from build123d import *

# Parameters (mm, degrees)
BOSS_EXTRUDE1_DEPTH      = 1.3
BOSS_EXTRUDE2_DEPTH      = 3.8
BOSS_EXTRUDE3_DEPTH      = 5.7
SKETCH4_R                = 0.5
CUT_EXTRUDE1_DEPTH       = 5.7
LPATTERN1_COUNT          = 6
LPATTERN1_PITCH          = 3
MIRROR1_COPY_1_SKETCH_R  = 0.5
MIRROR1_COPY_1_DEPTH     = 5.7
MIRROR1_COPY_2_SKETCH_R  = 0.5
MIRROR1_COPY_2_DEPTH     = 5.7
MIRROR1_COPY_3_SKETCH_R  = 0.5
MIRROR1_COPY_3_DEPTH     = 5.7
MIRROR1_COPY_4_SKETCH_R  = 0.5
MIRROR1_COPY_4_DEPTH     = 5.7
MIRROR1_COPY_5_SKETCH_R  = 0.5
MIRROR1_COPY_5_DEPTH     = 5.7
MIRROR2_COPY_1_SKETCH_R  = 0.5
MIRROR2_COPY_1_DEPTH     = 5.7
MIRROR2_COPY_2_SKETCH_R  = 0.5
MIRROR2_COPY_2_DEPTH     = 5.7
MIRROR2_COPY_3_SKETCH_R  = 0.5
MIRROR2_COPY_3_DEPTH     = 5.7
MIRROR2_COPY_4_SKETCH_R  = 0.5
MIRROR2_COPY_4_DEPTH     = 5.7
MIRROR2_COPY_5_SKETCH_R  = 0.5
MIRROR2_COPY_5_DEPTH     = 5.7
MIRROR2_COPY_6_SKETCH_R  = 0.5
MIRROR2_COPY_6_DEPTH     = 5.7
MIRROR2_COPY_7_SKETCH_R  = 0.5
MIRROR2_COPY_7_DEPTH     = 5.7
MIRROR2_COPY_8_SKETCH_R  = 0.5
MIRROR2_COPY_8_DEPTH     = 5.7
MIRROR2_COPY_9_SKETCH_R  = 0.5
MIRROR2_COPY_9_DEPTH     = 5.7
MIRROR2_COPY_10_SKETCH_R = 0.5
MIRROR2_COPY_10_DEPTH    = 5.7
MIRROR2_COPY_11_SKETCH_R = 0.5
MIRROR2_COPY_11_DEPTH    = 5.7
MIRROR2_COPY_12_SKETCH_R = 0.5
MIRROR2_COPY_12_DEPTH    = 5.7
MIRROR2_COPY_13_SKETCH_R = 0.5
MIRROR2_COPY_13_DEPTH    = 5.7
SKETCH5_R                = 1.55
CUT_EXTRUDE2_DEPTH       = 28.864942132


with BuildPart() as part:
    # Sketch1 → Boss-Extrude1 (new body)
    with BuildSketch(Plane.XY):
        with BuildLine():
            Line((-25.05, -6.25), (25.05, -6.25))
            ThreePointArc((25.05, -6.25), (26.110660172, -5.810660172), (26.55, -4.75))
            Line((26.55, -4.75), (26.55, 4.75))
            ThreePointArc((26.55, 4.75), (26.110660172, 5.810660172), (25.05, 6.25))
            Line((25.05, 6.25), (-25.05, 6.25))
            ThreePointArc((-25.05, 6.25), (-26.110660172, 5.810660172), (-26.55, 4.75))
            Line((-26.55, 4.75), (-26.55, -4.75))
            ThreePointArc((-26.55, -4.75), (-26.110660172, -5.810660172), (-25.05, -6.25))
        make_face()
    extrude(amount=BOSS_EXTRUDE1_DEPTH)

    # Sketch2 → Boss-Extrude2 (add)
    with BuildSketch(Plane(origin=(0, 0, 0), x_dir=(-1, 0, 0), z_dir=(0, 0, -1))):
        with BuildLine():
            Line((-18.7, -5.5), (18.7, -5.5))
            ThreePointArc((18.7, -5.5), (20.114213562, -4.914213562), (20.7, -3.5))
            Line((20.7, -3.5), (20.7, 3.5))
            ThreePointArc((20.7, 3.5), (20.114213562, 4.914213562), (18.7, 5.5))
            Line((18.7, 5.5), (-18.7, 5.5))
            ThreePointArc((-18.7, 5.5), (-20.114213562, 4.914213562), (-20.7, 3.5))
            Line((-20.7, 3.5), (-20.7, -3.5))
            ThreePointArc((-20.7, -3.5), (-20.114213562, -4.914213562), (-18.7, -5.5))
        make_face()
    extrude(amount=BOSS_EXTRUDE2_DEPTH)

    # Sketch3 → Boss-Extrude3 (add)
    with BuildSketch(Plane.XY.offset(1.3)):
        with BuildLine():
            Line((-17.25, -4.1), (17.25, -4.1))
            ThreePointArc((17.25, -4.1), (18.664213562, -3.514213562), (19.25, -2.1))
            Line((19.25, -2.1), (19.25, 2.1))
            ThreePointArc((19.25, 2.1), (18.664213562, 3.514213562), (17.25, 4.1))
            Line((17.25, 4.1), (-17.25, 4.1))
            ThreePointArc((-17.25, 4.1), (-18.664213562, 3.514213562), (-19.25, 2.1))
            Line((-19.25, 2.1), (-19.25, -2.1))
            ThreePointArc((-19.25, -2.1), (-18.664213562, -3.514213562), (-17.25, -4.1))
        make_face()
    extrude(amount=BOSS_EXTRUDE3_DEPTH)

    # Sketch4 → Cut-Extrude1 (cut)
    with BuildSketch(Plane.XY.offset(7)):
        with Locations((0, 2)):
            Circle(SKETCH4_R)
    cut_extrude1 = extrude(amount=-CUT_EXTRUDE1_DEPTH, mode=Mode.SUBTRACT)

    # LPattern1: Cut-Extrude1 ×6
    with Locations(*[(i * LPATTERN1_PITCH, 0, 0) for i in range(1, LPATTERN1_COUNT)]):
        add(cut_extrude1, mode=Mode.SUBTRACT)

    # Mirror1: Cut-Extrude1 across plane
    add(cut_extrude1.mirror(Plane.ZX), mode=Mode.SUBTRACT)

    # Mirror1 copy 1 sketch → Mirror1 copy 1 (cut)
    with BuildSketch(Plane(origin=(3, 0, 7), x_dir=(1, 0, 0), z_dir=(0, 0, 1))):
        with Locations((0, -2)):
            Circle(MIRROR1_COPY_1_SKETCH_R)
    extrude(amount=-MIRROR1_COPY_1_DEPTH, mode=Mode.SUBTRACT)

    # Mirror1 copy 2 sketch → Mirror1 copy 2 (cut)
    with BuildSketch(Plane(origin=(6, 0, 7), x_dir=(1, 0, 0), z_dir=(0, 0, 1))):
        with Locations((0, -2)):
            Circle(MIRROR1_COPY_2_SKETCH_R)
    extrude(amount=-MIRROR1_COPY_2_DEPTH, mode=Mode.SUBTRACT)

    # Mirror1 copy 3 sketch → Mirror1 copy 3 (cut)
    with BuildSketch(Plane(origin=(9, 0, 7), x_dir=(1, 0, 0), z_dir=(0, 0, 1))):
        with Locations((0, -2)):
            Circle(MIRROR1_COPY_3_SKETCH_R)
    extrude(amount=-MIRROR1_COPY_3_DEPTH, mode=Mode.SUBTRACT)

    # Mirror1 copy 4 sketch → Mirror1 copy 4 (cut)
    with BuildSketch(Plane(origin=(12, 0, 7), x_dir=(1, 0, 0), z_dir=(0, 0, 1))):
        with Locations((0, -2)):
            Circle(MIRROR1_COPY_4_SKETCH_R)
    extrude(amount=-MIRROR1_COPY_4_DEPTH, mode=Mode.SUBTRACT)

    # Mirror1 copy 5 sketch → Mirror1 copy 5 (cut)
    with BuildSketch(Plane(origin=(15, 0, 7), x_dir=(1, 0, 0), z_dir=(0, 0, 1))):
        with Locations((0, -2)):
            Circle(MIRROR1_COPY_5_SKETCH_R)
    extrude(amount=-MIRROR1_COPY_5_DEPTH, mode=Mode.SUBTRACT)

    # Mirror2 copy 1 sketch → Mirror2 copy 1 (cut)
    with BuildSketch(Plane(origin=(-3, 0, 7), x_dir=(-1, 0, 0), z_dir=(0, 0, 1))):
        with Locations((0, -2)):
            Circle(MIRROR2_COPY_1_SKETCH_R)
    extrude(amount=-MIRROR2_COPY_1_DEPTH, mode=Mode.SUBTRACT)

    # Mirror2 copy 2 sketch → Mirror2 copy 2 (cut)
    with BuildSketch(Plane(origin=(-6, 0, 7), x_dir=(-1, 0, 0), z_dir=(0, 0, 1))):
        with Locations((0, -2)):
            Circle(MIRROR2_COPY_2_SKETCH_R)
    extrude(amount=-MIRROR2_COPY_2_DEPTH, mode=Mode.SUBTRACT)

    # Mirror2 copy 3 sketch → Mirror2 copy 3 (cut)
    with BuildSketch(Plane(origin=(-9, 0, 7), x_dir=(-1, 0, 0), z_dir=(0, 0, 1))):
        with Locations((0, -2)):
            Circle(MIRROR2_COPY_3_SKETCH_R)
    extrude(amount=-MIRROR2_COPY_3_DEPTH, mode=Mode.SUBTRACT)

    # Mirror2 copy 4 sketch → Mirror2 copy 4 (cut)
    with BuildSketch(Plane(origin=(-12, 0, 7), x_dir=(-1, 0, 0), z_dir=(0, 0, 1))):
        with Locations((0, -2)):
            Circle(MIRROR2_COPY_4_SKETCH_R)
    extrude(amount=-MIRROR2_COPY_4_DEPTH, mode=Mode.SUBTRACT)

    # Mirror2 copy 5 sketch → Mirror2 copy 5 (cut)
    with BuildSketch(Plane(origin=(-15, 0, 7), x_dir=(-1, 0, 0), z_dir=(0, 0, 1))):
        with Locations((0, -2)):
            Circle(MIRROR2_COPY_5_SKETCH_R)
    extrude(amount=-MIRROR2_COPY_5_DEPTH, mode=Mode.SUBTRACT)

    # Mirror2 copy 6 sketch → Mirror2 copy 6 (cut)
    with BuildSketch(Plane(origin=(0, 0, 7), x_dir=(-1, 0, 0), z_dir=(0, 0, 1))):
        with Locations((0, -2)):
            Circle(MIRROR2_COPY_6_SKETCH_R)
    extrude(amount=-MIRROR2_COPY_6_DEPTH, mode=Mode.SUBTRACT)

    # Mirror2 copy 7 sketch → Mirror2 copy 7 (cut)
    with BuildSketch(Plane(origin=(0, 0, 7), x_dir=(-1, 0, 0), z_dir=(0, 0, 1))):
        with Locations((0, 2)):
            Circle(MIRROR2_COPY_7_SKETCH_R)
    extrude(amount=-MIRROR2_COPY_7_DEPTH, mode=Mode.SUBTRACT)

    # Mirror2 copy 8 sketch → Mirror2 copy 8 (cut)
    with BuildSketch(Plane(origin=(-3, 0, 7), x_dir=(-1, 0, 0), z_dir=(0, 0, 1))):
        with Locations((0, 2)):
            Circle(MIRROR2_COPY_8_SKETCH_R)
    extrude(amount=-MIRROR2_COPY_8_DEPTH, mode=Mode.SUBTRACT)

    # Mirror2 copy 9 sketch → Mirror2 copy 9 (cut)
    with BuildSketch(Plane(origin=(-6, 0, 7), x_dir=(-1, 0, 0), z_dir=(0, 0, 1))):
        with Locations((0, 2)):
            Circle(MIRROR2_COPY_9_SKETCH_R)
    extrude(amount=-MIRROR2_COPY_9_DEPTH, mode=Mode.SUBTRACT)

    # Mirror2 copy 10 sketch → Mirror2 copy 10 (cut)
    with BuildSketch(Plane(origin=(-9, 0, 7), x_dir=(-1, 0, 0), z_dir=(0, 0, 1))):
        with Locations((0, 2)):
            Circle(MIRROR2_COPY_10_SKETCH_R)
    extrude(amount=-MIRROR2_COPY_10_DEPTH, mode=Mode.SUBTRACT)

    # Mirror2 copy 11 sketch → Mirror2 copy 11 (cut)
    with BuildSketch(Plane(origin=(-12, 0, 7), x_dir=(-1, 0, 0), z_dir=(0, 0, 1))):
        with Locations((0, 2)):
            Circle(MIRROR2_COPY_11_SKETCH_R)
    extrude(amount=-MIRROR2_COPY_11_DEPTH, mode=Mode.SUBTRACT)

    # Mirror2 copy 12 sketch → Mirror2 copy 12 (cut)
    with BuildSketch(Plane(origin=(-15, 0, 7), x_dir=(-1, 0, 0), z_dir=(0, 0, 1))):
        with Locations((0, 2)):
            Circle(MIRROR2_COPY_12_SKETCH_R)
    extrude(amount=-MIRROR2_COPY_12_DEPTH, mode=Mode.SUBTRACT)

    # Mirror2 copy 13 sketch → Mirror2 copy 13 (cut)
    with BuildSketch(Plane(origin=(0, 0, 7), x_dir=(-1, 0, 0), z_dir=(0, 0, 1))):
        with Locations((0, -2)):
            Circle(MIRROR2_COPY_13_SKETCH_R)
    extrude(amount=-MIRROR2_COPY_13_DEPTH, mode=Mode.SUBTRACT)

    # Sketch5 → Cut-Extrude2 (cut, through all)
    with BuildSketch(Plane.XY.offset(1.3)):
        with Locations((23.75, 0)):
            Circle(SKETCH5_R)
    cut_extrude2 = extrude(amount=-CUT_EXTRUDE2_DEPTH, mode=Mode.SUBTRACT)

    # Mirror3: Cut-Extrude2 across plane
    add(cut_extrude2.mirror(Plane(origin=(0, 0, 0), x_dir=(0, 0, 1), z_dir=(1, 0, 0))), mode=Mode.SUBTRACT)


solid = part.part
Read the model definition and answer for the solid it produces. Units are mm, in the model's axes. A direction names the side the tool comes from. Round coordinates to 2 decimals unless told otherwise and drop trailing zeros. Loops run counter-clockwise (first coordinate to the right, second up) from the corner with the lowest first, then second, coordinate; pieces in that order, holes last.
Q1. Consider probe 1 along Y at (x, z) = (-15, 4.05); probe 2 along Z at (x, y) = (-22, -3); probe 3 along Y at (x, z) = (2, 6). Determine where each line is inside the solid, lowest interval first.
Q2. Section D-D on x = -18 is taken. Write down the section's boundary in (y, z), and give its area (3 significant figures).
Q3. Section B-B on y = 0 is taken. Write down the section's boundary in (x, z), and give its area (3 significant figures).
Q4. Section A-A on z = 4.75 is taken. Give the number of separate pieces and of enclosed holes in the cut face, and give its area (3 significant figures).
Q5. Determine the mould class of faces 4 (the face through (20.7, 0, -2)), 5 (the face through (-20.13, 4.9, -1.87)), 6 (the face through (2.6, 2.3, 4.2)) for opening direction X: released by +X, released by -X, zero draft, split by the parting line, or undercut.
Q6. Which of the six approach directions +Z, -Z, +X, -X, +Y, -Y give full straight-line access (tool end or side, diameter ignored) to faces 1 (the face through (18.68, 3.5, 4.11)), 2 (the face through (-12, 2, 1.3)), 3 (the face through (0, 6, 0))?
Q7. Section C-C on x = 13.5 is taken. Write down the section's boundary in (y, z).
Q8. Each of these flat-tipped pins is pushed along its axis until it touches: pin 1 (3 mm diameter, centred on x = -8.5, z = 4.5, fed in from +Y); pin 2 (3 mm diameter, centred on x = -4, z = -2, fed in from -Y); pin 3 (0.8 mm diameter, centred on x = 9, y = 2, fed in from +Z). Where does it stop, or does it pass through?
Output:
1. probe 1: y = -4.1 to -2.5, -1.5 to 1.5, 2.5 to 4.1
1. probe 2: z = 0 to 1.3
1. probe 3: y = -4.1 to 4.1
2. outline: (-6.25, 0) - (-5.5, 0) - (-5.5, -3.8) - (5.5, -3.8) - (5.5, 0) - (6.25, 0) - (6.25, 1.3) - (3.95, 1.3) - (3.95, 7) - (-3.95, 7) - (-3.95, 1.3) - (-6.25, 1.3) - close
2. area: 103 mm2
3. outline: (-26.55, 0) - (-25.3, 0) - (-25.3, 1.3) - (-26.55, 1.3) - close; (-22.2, 0) - (-20.7, 0) - (-20.7, -3.8) - (20.7, -3.8) - (20.7, 0) - (22.2, 0) - (22.2, 1.3) - (19.25, 1.3) - (19.25, 7) - (-19.25, 7) - (-19.25, 1.3) - (-22.2, 1.3) - close; (25.3, 0) - (26.55, 0) - (26.55, 1.3) - (25.3, 1.3) - close
3. area: 438 mm2
4. separate pieces: 1
4. enclosed holes: 22
4. area: 295 mm2
5. face 4: released by +X
5. face 5: released by -X
5. face 6: undercut
6. face 1: +Z, +X, +Y
6. face 2: +Z
6. face 3: -Z
7. outline: (-6.25, 0) - (-5.5, 0) - (-5.5, -3.8) - (5.5, -3.8) - (5.5, 0) - (6.25, 0) - (6.25, 1.3) - (4.1, 1.3) - (4.1, 7) - (-4.1, 7) - (-4.1, 1.3) - (-6.25, 1.3) - close
8. pin 1: stops at y = 4.1
8. pin 2: stops at y = -5.5
8. pin 3: stops at z = 1.3
